Autodesk Fusion 360 part; units mm, degrees
sketch "Sketch1" plane through (0, 0, 0) normal (0, 1, 0) x (1, 0, 0)
  line L0 (0, 0) -> (79, 0)
  line L1 (79, 0) -> (79, -170)
  line L2 (79, -170) -> (0, -170)
  line L3 (0, -170) -> (0, 0)
  line L4 (39.5, 0) -> (39.5, -169.9926) construction
  line L5 (49.5, -160) -> (29.5, -160) construction
  line L6 (29.5, -160) -> (29.5, -140) construction
  line L7 (29.5, -140) -> (49.5, -140) construction
  line L8 (49.5, -140) -> (49.5, -160) construction
  line L9 (49.5, -160) -> (29.5, -140) construction
  line L10 (29.5, -160) -> (49.5, -140) construction
  line L11 (55, -60.5) -> (24, -60.5) construction
  line L12 (24, -60.5) -> (24, -29.5) construction
  line L13 (24, -29.5) -> (55, -29.5) construction
  line L14 (55, -29.5) -> (55, -60.5) construction
  line L15 (55, -60.5) -> (24, -29.5) construction
  line L16 (24, -60.5) -> (55, -29.5) construction
  circle A0 centre (39.5, -45) radius 11.5
  point P0 (67.5, -110)
  point P1 (11.5, -110)
  point P2 (67.5, -90)
  point P3 (11.5, -90)
  point P4 (67.5, -70)
  point P5 (11.5, -70)
  point P6 (67.5, -50)
  point P7 (11.5, -50)
  point P8 (67.5, -30)
  point P9 (11.5, -30)
  point P10 (39.5, -150)
  point P11 (29.5, -140)
  point P12 (49.5, -140)
  point P13 (49.5, -160)
  point P14 (29.5, -160)
  point P15 (44.5, -150)
  point P16 (34.5, -150)
  point P17 (3.5, -167)
  point P18 (3.5, -161)
  point P19 (27.58, -101.35)
  point P20 (52.58, -101.35)
  point P21 (39.5, -45)
  point P22 (24, -29.5)
  point P23 (55, -29.5)
  point P24 (55, -60.5)
  point P25 (24, -60.5)
  point P26 (16, -19)
  point P27 (63, -19)
  point P28 (2.86, -19)
  point P29 (76.14, -19)
  dimension "d1" = 79
  dimension "d2" = 170
  dimension "d5" = 60
  dimension "d6" = 11.5
  dimension "d7" = 56
  dimension "d10" = 0
  dimension "d11" = 20
  dimension "d15" = 20
  dimension "d16" = 20
  dimension "d17" = 10
  dimension "d18" = 10
  dimension "d19" = 5
  dimension "d20" = 6
  dimension "d21" = 3.5
  dimension "d22" = 3
  dimension "d23" = 25
  dimension "d24" = 68.65
  dimension "d25" = 11.92
  dimension "d26" = 31
  dimension "d27" = 31
  dimension "d28" = 29.5
  dimension "d29" = 24
  dimension "d31" = 16
  dimension "d32" = 16
  dimension "d33" = 19
  dimension "d34" = 13.14
  dimension "d35" = 13.14
  dimension "d36" = 19
  dimension "d42" = 23
extrude "Extrude2" add sketch "Sketch1" against normal blind 6.41
hole "Hole2" at (3.5, 0, 161) direction (0, -1, 0) diameter 2 end through all counterbore diameter 4.4 counterbore depth 2
hole "Hole3" at (3.5, 0, 167) direction (0, -1, 0) diameter 2 end through all counterbore diameter 4.4 counterbore depth 2
sketch "Sketch2" plane through (0, -6.41, 0) normal (0, -1, 0) x (1, 0, 0)
  circle A0 centre (3.5, 167) radius 1
  circle A1 centre (3.5, 161) radius 1
  circle A2 centre (39.5, 45) radius 11.5
  line L0 (79, 170) -> (0, 170)
  line L1 (0, 170) -> (0, 0)
  line L2 (0, 0) -> (79, 0)
  line L3 (79, 0) -> (79, 170)
  line L4 (49.5, 140) -> (49.5, 160)
  point P0 (44.5, 150)
  point P1 (34.5, 150)
  dimension "d55" = 5
  dimension "d56" = 10
hole "Hole4" at (34.5, -6.41, 150) direction (0, 1, 0) diameter 2 end through all counterbore diameter 4.4 counterbore depth 2
hole "Hole5" at (44.5, -6.41, 150) direction (0, 1, 0) diameter 2 end through all counterbore diameter 4.4 counterbore depth 2
hole "Hole6" at (29.5, 0, 140) direction (0, -1, 0) diameter 3.4 end through all counterbore diameter 6.5 counterbore depth 3
hole "Hole7" at (49.5, 0, 140) direction (0, -1, 0) diameter 3.4 end through all counterbore diameter 6.5 counterbore depth 3
hole "Hole8" at (29.5, 0, 160) direction (0, -1, 0) diameter 3.4 end through all counterbore diameter 6.5 counterbore depth 3
hole "Hole9" at (49.5, 0, 160) direction (0, -1, 0) diameter 3.4 end through all counterbore diameter 6.5 counterbore depth 3
hole "Hole10" at (27.58, 0, 101.35) direction (0, -1, 0) diameter 3.4 end through all counterbore diameter 6.5 counterbore depth 3
hole "Hole11" at (52.58, 0, 101.35) direction (0, -1, 0) diameter 3.4 end through all counterbore diameter 6.5 counterbore depth 3
hole "Hole12" at (24, 0, 29.5) direction (0, -1, 0) diameter 3.4 end through all counterbore diameter 6.5 counterbore depth 3
hole "Hole13" at (55, 0, 29.5) direction (0, -1, 0) diameter 3.4 end through all counterbore diameter 6.5 counterbore depth 3
hole "Hole14" at (55, 0, 60.5) direction (0, -1, 0) diameter 3.4 end through all counterbore diameter 6.5 counterbore depth 3
hole "Hole15" at (24, 0, 60.5) direction (0, -1, 0) diameter 3.4 end through all counterbore diameter 6.5 counterbore depth 3
hole "Hole16" at (11.5, 0, 110) direction (0, -1, 0) diameter 2.5 end through all
hole "Hole17" at (11.5, 0, 90) direction (0, -1, 0) diameter 2.5 end through all
hole "Hole18" at (11.5, 0, 70) direction (0, -1, 0) diameter 2.5 end through all
hole "Hole19" at (11.5, 0, 50) direction (0, -1, 0) diameter 2.5 end through all
hole "Hole20" at (11.5, 0, 30) direction (0, -1, 0) diameter 2.5 end through all
hole "Hole21" at (67.5, 0, 110) direction (0, -1, 0) diameter 2.5 end through all
hole "Hole22" at (67.5, 0, 90) direction (0, -1, 0) diameter 2.5 end through all
hole "Hole23" at (67.5, 0, 70) direction (0, -1, 0) diameter 2.5 end through all
hole "Hole24" at (67.5, 0, 50) direction (0, -1, 0) diameter 2.5 end through all
hole "Hole25" at (67.5, 0, 30) direction (0, -1, 0) diameter 2.5 end through all
hole "Hole26" at (16, 0, 19) direction (0, -1, 0) diameter 2.5 end through all
hole "Hole27" at (63, 0, 19) direction (0, -1, 0) diameter 2.5 end through all
hole "Hole28" at (2.86, 0, 19) direction (0, -1, 0) diameter 2.8 end through all
hole "Hole29" at (76.14, 0, 19) direction (0, -1, 0) diameter 2.8 end through all
sketch "TopHolesSketch" plane through (0, 0, 0) normal (0, 0, -1) x (-1, 0, 0)
  line L0 (0, 0) -> (-79, 0)
  line L1 (-79, 0) -> (-79, -6.41)
  line L2 (-79, -6.41) -> (0, -6.41)
  line L3 (0, -6.41) -> (0, 0)
  line L4 (0, -3.205) -> (-79, -3.205) construction
  point P0 (-14, -3.205)
  point P1 (-31, -3.205)
  point P2 (-48, -3.205)
  point P3 (-65, -3.205)
  dimension "d159" = 14
  dimension "d162" = -17
  dimension "d163" = 0
hole "Hole30" at (14, -3.205, 0) direction (0, 0, 1) diameter 2.5 depth 10 tip angle 118
pattern_linear "R-Pattern1" count 4 spacing 17 along (1, 0, 0) of "Hole30"
sketch "Sketch4" plane through (0, 0, 0) normal (-1, 0, 0) x (0, 0, 1)
  line L0 (170, 0) -> (0, 0)
  line L1 (0, 0) -> (0, -6.41)
  line L2 (0, -6.41) -> (170, -6.41)
  line L3 (170, -6.41) -> (170, 0)
  line L4 (0, -3.205) -> (170, -3.205) construction
  point P0 (6, -3.205)
  point P1 (25, -3.205)
  point P2 (44, -3.205)
  point P3 (63, -3.205)
  point P4 (82, -3.205)
  point P5 (101, -3.205)
  point P6 (120, -3.205)
  point P7 (139, -3.205)
  point P8 (158, -3.205)
  dimension "d171" = 6
  dimension "d174" = 19
  dimension "d175" = 0
sketch "Sketch5" plane through (79, 0, 0) normal (1, 0, 0) x (0, 0, -1)
  line L0 (0, 0) -> (-170, 0)
  line L1 (-170, 0) -> (-170, -6.41)
  line L2 (-170, -6.41) -> (0, -6.41)
  line L3 (0, -6.41) -> (0, 0)
  line L4 (0, -3.205) -> (-170, -3.205) construction
  point P0 (-6, -3.205)
  point P1 (-25, -3.205)
  point P2 (-44, -3.205)
  point P3 (-63, -3.205)
  point P4 (-82, -3.205)
  point P5 (-101, -3.205)
  point P6 (-120, -3.205)
  point P7 (-139, -3.205)
  point P8 (-158, -3.205)
  dimension "d176" = 6
  dimension "d179" = -19
  dimension "d180" = 0
hole "Hole31" at (79, -3.205, 6) direction (-1, 0, 0) diameter 2.5 depth 10 tip angle 118
pattern_linear "R-Pattern2" count 1 spacing 19 along (0, -1, 0) count 9 spacing 19 along (0, 0, 1) of "Hole31"
hole "Hole32" at (0, -3.205, 6) direction (1, 0, 0) diameter 2.5 depth 10 tip angle 118
pattern_linear "R-Pattern3" count 1 spacing 0 along (0, -1, 0) count 9 spacing 19 along (0, 0, 1) of "Hole32"
Part model, mm, in its own coordinate system. A direction names the side the tool comes from. Round coordinates to 2 decimals unless told otherwise and drop trailing zeros. Loops run counter-clockwise (first coordinate to the right, second up) from the corner with the lowest first, then second, coordinate; pieces in that order, holes last.
1. 3-axis set-ups, long thin cutter, end or side, ignore diameter. For faces 4 (the face through (23.93, -4.73, 58.8)), 5 (the face through (50.745, -1.521, 163.002)): which of +Z, -Z, +X, -X, +Y, -Y reach the whole face in a straight line?
Solutions:
face 4: +Y, -Y
face 5: +Y
2. Slice it at A-A (x = 40). Give the cut face in (y, z), and give its area (3 significant figures).
Solutions:
outline: (-6.41, 0) - (0, 0) - (0, 33.51) - (-6.41, 33.51) - close; (-6.41, 56.49) - (0, 56.49) - (0, 170) - (-6.41, 170) - close
area: 942 mm2
3. Drill centre lines: line 1 along Z through (x, y) = (24, -5.3); line 2 along X through (y, z) = (-1.4, 150); line 3 along Z through (x, y) = (49, -2). Where is each one in solid material? Low to high.
Solutions:
line 1: z = 0 to 27.8, 31.2 to 58.8, 62.2 to 170
line 2: x = 0 to 33.5, 35.5 to 43.5, 45.5 to 79
line 3: z = 0 to 38.52, 51.48 to 136.79, 143.21 to 156.79, 163.21 to 170
4. Two-plate mould, pull along Z, no slides. Class faces 1 (the face through (40, -3, 170)), 2 (the face through (45.839, -5.396, 151.746)), 3 (the face through (39, -3, 0)): pulls with the +Z half, pulls with the -Z half, needs draft (parallel to the pull), parting line crosses it, or undercut.
Solutions:
face 1: pulls with the +Z half
face 2: undercut
face 3: pulls with the -Z half
5. Slice it at B-B (z = 37). Give the cut face in (x, y).
Solutions:
outline: (0, -6.41) - (31.24, -6.41) - (31.24, 0) - (0, 0) - close; (47.76, -6.41) - (79, -6.41) - (79, 0) - (47.76, 0) - close
6. Flat gauge pins, fed straight in: pin 1 (6 mm diameter, centred on x = 24, z = 60.5, fed in from +Y); pin 2 (5 mm diameter, centred on x = 13, z = 118, fed in from +Y). Where does each tip first touch, or does it go through?
Solutions:
pin 1: stops at y = -3
pin 2: stops at y = 0
